Part model, mm, in its own coordinate system. A direction names the side the tool comes from. Coordinates: 2 decimals unless noted, no trailing zeros. Write each loop counter-clockwise with the first axis right and the second up, starting at its lowest first coordinate (ties: lowest second). Pieces come first, ordered by that corner, then holes. Notation, with made-up numbers: (26.25, 48) -> (68.25, 48) arc R13 ccw to (68.25, 61) -> close; hole circle Ø4 at (-38, 2). An arc over 180 degrees is marked (long way). Write item = value, one per line. Start each with the question number.
Q1. Probe line 1 (Z direction, x = -63.5, y = -6.5); line 2 (Z direction, x = -51, y = -6); line 3 (X direction, y = -13, z = -48). List the from-to ranges inside material, lowest first.
Q2. Band-saw the part on D-D, the plane z = -17.5. List the corners of the cut face in (x, y), plus the area to 3 significant figures.
Q3. Band-saw the part on B-B, the plane y = -21. List the corners of the cut face in (x, z), plus the area to 3 significant figures.
Q4. Pull direction X, two halves, no side cores. Call faces 4 (the flat face through (-61.566, -21, -28)), 5 (the flat face through (-63, -21, -56.524)), 6 (the flat face through (-64.566, -21, -27)), 7 (the cylindrical face through (-56.404, -29.044, 2.49)): released by +X, released by -X, zero draft, split by the parting line, or undercut.
Q5. Band-saw the part on A-A, the plane y = -35.5. List the corners of the cut face in (x, z).
Q6. Pin check, flat tips, straight feed: P1, Ø2, axis at x = -54.5, y = -26, coming from the -Z side; P2, Ø2, axis at y = -8, z = -38.5, coming from the +X side; P3, Ø3, axis at x = -41.9, y = -28.7, coming from the +Z side. Stop position of each tip, or through.
Q7. Band-saw the part on C-C, the plane x = -46.25. List the corners of the cut face in (y, z).
Q8. Tool access for faces 1 (the flat face through (-42, -21, 1.476)), 2 (the cylindrical face through (-63.09, -6.24, -49.54)), 3 (the cylindrical face through (-57.31, -20.66, 13.34)): list every direction of +Z, -Z, +X, -X, +Y, -Y with a clear straight run to the whole face (end or side of a thin tool).
from build123d import *

# Parameters (mm, degrees)
F0_W      = 3
F0_H      = 60
F1_DEPTH  = 42
F2_W      = 30
F2_H      = 2
F3_DEPTH  = 42
F4_R      = 7.5
F4_W      = 30
F4_H      = 42
F5_DEPTH  = 2
F6_R      = 7.75
F6_R_2    = 6.75
F7_DEPTH  = 20
F9_R      = 2
F10_DEPTH = 25
F11_DEPTH = 25
F8_R      = 0.9
F12_DEPTH = 25


with BuildPart() as f1:
    # F0 (on Front) → F1 (new body)
    with BuildSketch(Plane.XZ):
        with Locations((-63.065696, -26.523725)):
            Rectangle(F0_W, F0_H)
    extrude(amount=F1_DEPTH)

    # F2 (on Front) → F3 (join)
    with BuildSketch(Plane.XZ):
        with Locations((-49.565696, 2.476275)):
            Rectangle(F2_W, F2_H)
    extrude(amount=F3_DEPTH)

    # F4 (on face) → F5 (join)
    with BuildSketch(Plane.XY.offset(3.476275)):
        with Locations((-43.565696, -21)):
            Circle(F4_R)
        with Locations((-49.565696, -21)):
            Rectangle(F4_W, F4_H)
        with Locations((-43.565696, -21)):
            Circle(F4_R, mode=Mode.SUBTRACT)
    extrude(amount=-F5_DEPTH)

    # F6 (on face) → F7 (join)
    with BuildSketch(Plane.XY.offset(3.476275)):
        with Locations((-49.565696, -21)):
            Circle(F6_R)
        with Locations((-49.565696, -21)):
            Circle(F6_R_2, mode=Mode.SUBTRACT)
    extrude(amount=F7_DEPTH)

    # F9 (on face) → F10 (cut)
    with BuildSketch(Plane(origin=(-64.565696, 0, 0), x_dir=(0, -1, 0), z_dir=(-1, 0, 0))):
        with Locations((35.5, -51.523725)):
            Circle(F9_R)
        with Locations((6.5, -51.523725)):
            Circle(F9_R)
    extrude(amount=-F10_DEPTH, mode=Mode.SUBTRACT)

    # F6 (on face) → F11 (cut)
    with BuildSketch(Plane.XY.offset(3.476275)):
        with Locations((-49.565696, -21)):
            Circle(F6_R_2)
    extrude(amount=-F11_DEPTH, mode=Mode.SUBTRACT)

    # F8 (on face) → F12 (cut)
    with BuildSketch(Plane.XY.offset(3.476275)):
        with Locations((-57.235696, -28.698958)):
            Circle(F8_R)
        with Locations((-41.895696, -28.698951)):
            Circle(F8_R)
    extrude(amount=-F12_DEPTH, mode=Mode.SUBTRACT)


solid = f1.part
Ans:
q1.line_1 = -56.52 to -53.52, -49.52 to 3.48
q1.line_2 = 1.48 to 3.48
q1.line_3 = -64.57 to -61.57
q2.outline = (-64.57, -42) -> (-61.57, -42) -> (-61.57, 0) -> (-64.57, 0) -> close
q2.area = 126 mm2
q3.outline = (-64.57, -56.52) -> (-61.57, -56.52) -> (-61.57, 1.48) -> (-56.32, 1.48) -> (-56.32, 23.48) -> (-57.32, 23.48) -> (-57.32, 3.48) -> (-64.57, 3.48) -> close; (-42.82, 1.48) -> (-34.57, 1.48) -> (-34.57, 3.48) -> (-41.82, 3.48) -> (-41.82, 23.48) -> (-42.82, 23.48) -> close
q3.area = 247 mm2
q4.face_4 = released by +X
q4.face_5 = zero draft
q4.face_6 = released by -X
q4.face_7 = undercut
q5.outline = (-64.57, -56.52) -> (-61.57, -56.52) -> (-61.57, -53.52) -> (-64.57, -53.52) -> close; (-64.57, -49.52) -> (-61.57, -49.52) -> (-61.57, 1.48) -> (-34.57, 1.48) -> (-34.57, 3.48) -> (-64.57, 3.48) -> close
q6.P1 = 1.48
q6.P2 = -61.57
q6.P3 = 3.48
q7.outline = (-42, 1.48) -> (-26.88, 1.48) -> (-26.88, 23.48) -> (-28, 23.48) -> (-28, 3.48) -> (-42, 3.48) -> close; (-15.12, 1.48) -> (0, 1.48) -> (0, 3.48) -> (-14, 3.48) -> (-14, 23.48) -> (-15.12, 23.48) -> close
q8.face_1 = -Z, +X, +Y, -Y
q8.face_2 = +X, -X
q8.face_3 = +Z
